```python
from build123d import *

# Parameters (mm, degrees)
SKETCH1_W           = 26.5
SKETCH1_H           = 15.8
SKETCH1_W_2         = 22.5
SKETCH1_H_2         = 11.8
BOSS_EXTRUDE1_DEPTH = 3
SKETCH2_W           = 26.5
SKETCH2_H           = 15.8
SKETCH2_R           = 1.5
BOSS_EXTRUDE2_DEPTH = 3
SKETCH3_R           = 3
CUT_EXTRUDE1_DEPTH  = 2


with BuildPart() as part:
    # Sketch1 → Boss-Extrude1 (new body)
    with BuildSketch(Plane(origin=(0, 0, 0), x_dir=(0, 0, -1), z_dir=(1, 0, 0))):
        with Locations((-5.35, 0)):
            Rectangle(SKETCH1_W, SKETCH1_H)
        with Locations((-5.35, 0)):
            Rectangle(SKETCH1_W_2, SKETCH1_H_2, mode=Mode.SUBTRACT)
    extrude(amount=BOSS_EXTRUDE1_DEPTH)

    # Sketch2 → Boss-Extrude2 (add)
    with BuildSketch(Plane(origin=(3, 0, 0), x_dir=(0, 0, -1), z_dir=(1, 0, 0))):
        with Locations((-5.35, 0)):
            Rectangle(SKETCH2_W, SKETCH2_H)
        Circle(SKETCH2_R, mode=Mode.SUBTRACT)
    extrude(amount=BOSS_EXTRUDE2_DEPTH)

    # Sketch3 → Cut-Extrude1 (cut)
    with BuildSketch(Plane.ZY.offset(-3)):
        Circle(SKETCH3_R)
    extrude(amount=-CUT_EXTRUDE1_DEPTH, mode=Mode.SUBTRACT)


solid = part.part
```
The model under review builds one solid part; all positions refer to its coordinate system, in mm. A direction names the side the tool comes from. Round coordinates to 2 decimals unless told otherwise and drop trailing zeros. Order: outer loops, then holes, each group sorted by start corner. A loop starts at its lowest first (then second) coordinate and runs counter-clockwise, first axis right, second up. Notation, with made-up numbers: (49, -16) -> (79, -16) arc R35 cw to (79, 17) -> close; hole circle Ø9 at (63, -32). An arc over 180 degrees is marked (long way). Use a Markdown table: item, result.
Q1. We need section B-B on x = 0.9. Write out the cut boundary in (y, z), then the cut area to 3 significant figures.
Values:
| item | result |
|---|---|
| outline | (-7.9, -7.9) -> (7.9, -7.9) -> (7.9, 18.6) -> (-7.9, 18.6) -> close; hole (-5.9, -5.9) -> (5.9, -5.9) -> (5.9, 16.6) -> (-5.9, 16.6) -> close |
| area | 153 mm^2 |
Q2. Tool access review of faces 1 (the flat face through (0, -7, 6)), 2 (the cylindrical face through (4, 0, -3)): name each direction out of +Z, -Z, +X, -X, +Y, -Y from which nothing blocks a thin tool from reaching the whole face with its end or side.
Values:
| item | result |
|---|---|
| face 1 | +Z, -Z, -X, +Y, -Y |
| face 2 | -X |
Q3. We need section A-A on z = 0. Write out the cut boundary in (x, y), then the cut area to 3 significant figures.
Values:
| item | result |
|---|---|
| outline | (0, -7.9) -> (6, -7.9) -> (6, -1.5) -> (5, -1.5) -> (5, -3) -> (3, -3) -> (3, -5.9) -> (0, -5.9) -> close; (0, 5.9) -> (3, 5.9) -> (3, 3) -> (5, 3) -> (5, 1.5) -> (6, 1.5) -> (6, 7.9) -> (0, 7.9) -> close |
| area | 44.4 mm^2 |
Q4. We need section C-C on y = 0. Write out the cut boundary in (x, z), then the cut area to 3 significant figures.
Values:
| item | result |
|---|---|
| outline | (0, -7.9) -> (6, -7.9) -> (6, -1.5) -> (5, -1.5) -> (5, -3) -> (3, -3) -> (3, -5.9) -> (0, -5.9) -> close; (0, 16.6) -> (3, 16.6) -> (3, 3) -> (5, 3) -> (5, 1.5) -> (6, 1.5) -> (6, 18.6) -> (0, 18.6) -> close |
| area | 76.5 mm^2 |
Q5. Mouldability with a two-part tool opening along Y and no side actions: class faces 3 (the flat face through (3, 0, -7.9)), 4 (the cylindrical face through (5.49, 0.07, 1.5)), 5 (the flat face through (3, 7.9, 6)), 6 (the flat face through (1, 0, 16.6)) as +Y half, -Y half, draft (parallel to the pull), parting line (faces both ways), or undercut.
Values:
| item | result |
|---|---|
| face 3 | draft |
| face 4 | undercut |
| face 5 | +Y half |
| face 6 | undercut |
Q6. We need section D-D on y = 5. Write out the cut boundary in (x, z).
Values:
| item | result |
|---|---|
| outline | (0, -7.9) -> (6, -7.9) -> (6, 18.6) -> (0, 18.6) -> (0, 16.6) -> (3, 16.6) -> (3, -5.9) -> (0, -5.9) -> close |
Q7. For line 1 (Y direction, x = 2.75, z = 3.5); line 2 (Y direction, x = 5.3, z = 0); line 3 (Z direction, x = 5.4, y = 0), list the stretches that pass through material, from the lowest coordinate up.
Values:
| item | result |
|---|---|
| line 1 | y = -7.9 to -5.9, 5.9 to 7.9 |
| line 2 | y = -7.9 to -1.5, 1.5 to 7.9 |
| line 3 | z = -7.9 to -1.5, 1.5 to 18.6 |
Q8. Clearance check with flat-ended pins moving along their axes: P1, Ø3.5, axis at y = 0, z = 0, coming from the -X side; P2, Ø6, axis at y = 1, z = 1, coming from the -X side; P3, Ø2.5, axis at y = 0, z = 0, coming from the +X side. State where each tip first meets the part, or that it passes through.
Values:
| item | result |
|---|---|
| P1 | stops at x = 5 |
| P2 | stops at x = 3 |
| P3 | passes through |
